Here's how the part is built. I have some questions about the finished solid (model axes, mm). Give positions to 0.01 mm unless a question says otherwise; leave off trailing zeros. Write each loop counter-clockwise with the first axis right and the second up, starting at its lowest first coordinate (ties: lowest second). Pieces come first, ordered by that corner, then holes. Notation, with made-up numbers: (38.5, 76) - (89.5, 76) arc R23 ccw to (89.5, 108) - close; hole circle Ø11 at (-9, 37). An arc over 180 degrees is marked (long way). Use one line per item in the form item = value. Start each with the question number.
from build123d import *

# Parameters (mm, degrees)
SKETCH1_W             = 110
SKETCH1_H             = 46
BOSS_EXTRUDE1_DEPTH   = 6.35
M6_CLEARANCE_HOLE1_D  = 6.4
SKETCH5_R             = 5.5
CUT_EXTRUDE1_DEPTH    = 7.35
SKETCH7_R             = 4.5
CUT_EXTRUDE2_DEPTH    = 7.35
FILLET1_R             = 5
F_8_32_TAPPED_HOLE1_D = 3.4544
F_8_CLEARANCE_HOLE1_D = 4.3053
F_8_32_TAPPED_HOLE2_D = 3.4544


with BuildPart() as part:
    # Sketch1 → Boss-Extrude1 (new body)
    with BuildSketch(Plane.XY):
        Rectangle(SKETCH1_W, SKETCH1_H)
    extrude(amount=BOSS_EXTRUDE1_DEPTH)

    # M6 Clearance Hole1 (through all)
    with Locations(Plane(origin=(0, 0, 0), x_dir=(-1, 0, 0), z_dir=(0, 0, -1))):
        with Locations((-35, 10), (-35, -10), (35, -10), (35, 10)):
            Hole(M6_CLEARANCE_HOLE1_D / 2)

    # Sketch5 → Cut-Extrude1 (cut, through all)
    with BuildSketch(Plane(origin=(0, 0, 0), x_dir=(-1, 0, 0), z_dir=(0, 0, -1))):
        with Locations((-10, -5)):
            Circle(SKETCH5_R)
        with Locations((10, -5)):
            Circle(SKETCH5_R)
    extrude(amount=-CUT_EXTRUDE1_DEPTH, mode=Mode.SUBTRACT)

    # Sketch7 → Cut-Extrude2 (cut, through all)
    with BuildSketch(Plane(origin=(0, 0, 0), x_dir=(-1, 0, 0), z_dir=(0, 0, -1))):
        with Locations((-23, 9)):
            Circle(SKETCH7_R)
        with Locations((-23, -9)):
            Circle(SKETCH7_R)
        with Locations((23, -9)):
            Circle(SKETCH7_R)
        with Locations((23, 9)):
            Circle(SKETCH7_R)
        with Locations((-47, 9)):
            Circle(SKETCH7_R)
        with Locations((-47, -9)):
            Circle(SKETCH7_R)
        with Locations((47, 9)):
            Circle(SKETCH7_R)
        with Locations((47, -9)):
            Circle(SKETCH7_R)
    extrude(amount=-CUT_EXTRUDE2_DEPTH, mode=Mode.SUBTRACT)

    # Fillet1
    fillet1_edges = [part.edges().sort_by_distance(p)[0] for p in [
        (-55, -23, 3.175),
        (-55, 23, 3.175),
        (55, 23, 3.175),
        (55, -23, 3.175),
    ]]
    fillet(fillet1_edges, radius=FILLET1_R)

    # #8-32 Tapped Hole1 (through all)
    with Locations(Plane(origin=(0, 0, 0), x_dir=(-1, 0, 0), z_dir=(0, 0, -1))):
        with Locations((-23, 19), (23, 19), (23, -19), (-23, -19)):
            Hole(F_8_32_TAPPED_HOLE1_D / 2)

    # #8 Clearance Hole1 (through all)
    with Locations(Plane(origin=(0, 0, 0), x_dir=(-1, 0, 0), z_dir=(0, 0, -1))):
        with Locations((-50, 19), (-50, -19), (50, -19), (50, 19)):
            Hole(F_8_CLEARANCE_HOLE1_D / 2)

    # #8-32 Tapped Hole2 (through all)
    with Locations(Plane(origin=(0, 0, 0), x_dir=(-1, 0, 0), z_dir=(0, 0, -1))):
        with Locations((-11.5, 10), (11.5, 10), (11.5, -18), (-11.5, -18), (-15, -14), (15, -14), (15, 16), (-15, 16)):
            Hole(F_8_32_TAPPED_HOLE2_D / 2)


solid = part.part
1. We'd pull the mould along Y, two halves only. Please class faces 1 (the face through (-50.28, -16.866, 3.219)), 2 (the face through (-1, -23, 3)), 3 (the face through (53, 22, 3)), 4 (the face through (-1, 0, 6.35)): pulls with the +Y half, pulls with the -Y half, needs draft (parallel to the pull), parting line crosses it, or undercut.
2. I want a section at B-B, the plane x = -35. List the corners of the cut face in (y, z) for me.
3. I want a section at C-C, the plane y = 19. List the corners of the cut face in (x, z) for me.
4. I want a section at A-A, the plane x = -23. List the corners of the cut face in (y, z) for me, then the cut area to 3 significant figures.
5. I want a section at D-D, the plane x = 7.5. List the corners of the cut face in (y, z) for me.
6. Please list where these lines run through material, in increasing order: line 1 (Y direction, x = -35, z = 2); line 2 (Y direction, x = 23, z = 2.75); line 3 (Y direction, x = -21, z = 3.5).
Result sheet:
q1.face_1 = undercut
q1.face_2 = pulls with the -Y half
q1.face_3 = pulls with the +Y half
q1.face_4 = needs draft
q2.outline = (-23, 0) - (-13.2, 0) - (-13.2, 6.35) - (-23, 6.35) - close; (-6.8, 0) - (6.8, 0) - (6.8, 6.35) - (-6.8, 6.35) - close; (13.2, 0) - (23, 0) - (23, 6.35) - (13.2, 6.35) - close
q3.outline = (-54.9, 0) - (-52.15, 0) - (-52.15, 6.35) - (-54.9, 6.35) - close; (-47.85, 0) - (-24.73, 0) - (-24.73, 6.35) - (-47.85, 6.35) - close; (-21.27, 0) - (21.27, 0) - (21.27, 6.35) - (-21.27, 6.35) - close; (24.73, 0) - (47.85, 0) - (47.85, 6.35) - (24.73, 6.35) - close; (52.15, 0) - (54.9, 0) - (54.9, 6.35) - (52.15, 6.35) - close
q4.outline = (-23, 0) - (-20.73, 0) - (-20.73, 6.35) - (-23, 6.35) - close; (-17.27, 0) - (-13.5, 0) - (-13.5, 6.35) - (-17.27, 6.35) - close; (-4.5, 0) - (4.5, 0) - (4.5, 6.35) - (-4.5, 6.35) - close; (13.5, 0) - (17.27, 0) - (17.27, 6.35) - (13.5, 6.35) - close; (20.73, 0) - (23, 0) - (23, 6.35) - (20.73, 6.35) - close
q4.area = 134 mm2
q5.outline = (-23, 0) - (-9.9, 0) - (-9.9, 6.35) - (-23, 6.35) - close; (-0.1, 0) - (23, 0) - (23, 6.35) - (-0.1, 6.35) - close
q6.line_1 = -23 to -13.2, -6.8 to 6.8, 13.2 to 23
q6.line_2 = -23 to -20.73, -17.27 to -13.5, -4.5 to 4.5, 13.5 to 17.27, 20.73 to 23
q6.line_3 = -23 to -13.03, -4.97 to 4.97, 13.03 to 23
